Input: part model. Units: mm. Frame: model coordinates. Face numbers are marked on the shaded views. A direction names the side the tool comes from. Round coordinates to 2 decimals unless told otherwise and drop trailing zeros. Write each loop counter-clockwise with the first axis right and the second up, starting at its lowest first coordinate (ties: lowest second). Pieces come first, ordered by that corner, then holes. Notation, with made-up numbers: (84.25, -17) - (108.25, -17) arc R25 ccw to (108.25, 21) - close; hole circle Ø1 at (59, 34). An arc over 180 degrees is marked (long way). One line per item, written item: value. Start each with the question number.
```python
from build123d import *

# Parameters (mm, degrees)
F1_DEPTH = 12.7
F2_W     = 22.225
F2_H     = 12.7
F3_DEPTH = 10.16
F4_R     = 5.08
F5_R     = 3.81
F6_W     = 2.032
F6_H     = 1.016
F7_DEPTH = 1.905
F8_R     = 0.50799


# Not quite as in the source:
# - a fillet or chamfer is up to 0.001 mm smaller than in the source, because OpenCascade refuses the exact size


with BuildPart() as f1:
    # F0 (on Front) → F1 (new body)
    with BuildSketch(Plane.XZ):
        with BuildLine():
            Line((-12.7675240695, 14.3095031442), (-12.7675240695, -11.0904968558))
            Line((-12.7675240695, -11.0904968558), (9.4574759305, -11.0904968558))
            Line((9.4574759305, -11.0904968558), (9.4574759305, 14.3095031442))
            ThreePointArc((9.4574759305, 14.3095031442), (-1.6550240695, 3.1970031442), (-12.7675240695, 14.3095031442))
        make_face()
        with BuildLine():
            ThreePointArc((9.4574759305, 14.3095031442), (-1.6550240695, 25.4220031442), (-12.7675240695, 14.3095031442))
            ThreePointArc((-12.7675240695, 14.3095031442), (-1.6550240695, 3.1970031442), (9.4574759305, 14.3095031442))
        make_face()
    extrude(amount=F1_DEPTH)

    # F2 (on face) → F3 (join)
    with BuildSketch(Plane.XZ.offset(12.7)):
        with Locations((-1.6550240695, -4.7404968558)):
            Rectangle(F2_W, F2_H)
    extrude(amount=F3_DEPTH)

    # F4
    f4_edges = [f1.edges().sort_by_distance(p)[0] for p in [
        (9.457476, -12.7, 7.959503),
        (-12.767524, -17.78, 1.609503),
        (9.457476, -17.78, 1.609503),
    ]]
    fillet(f4_edges, radius=F4_R)

    # F5
    f5_edges = [f1.edges().sort_by_distance(p)[0] for p in [
        (-12.767524, -11.43, -11.090497),
        (9.457476, -11.43, -11.090497),
    ]]
    fillet(f5_edges, radius=F5_R)

    # F6 (on face) → F7 (join)
    with BuildSketch(Plane(origin=(0, 0, 0), x_dir=(-1, 0, 0), z_dir=(0, 1, 0))):
        with Locations((1.6550240695, 14.3095031442)):
            Rectangle(F6_W, F6_H)
    extrude(amount=F7_DEPTH)

    # F8 (radius 0.508 in the source; OpenCascade refuses exactly that, so slightly less here)
    f8_edges = [f1.edges().sort_by_distance(p)[0] for p in [
        (-0.639024, 0.9525, 14.817503),
        (-0.639024, 0.9525, 13.801503),
        (-2.671024, 0.9525, 13.801503),
        (-2.671024, 0.9525, 14.817503),
    ]]
    fillet(f8_edges, radius=F8_R)


solid = f1.part
```
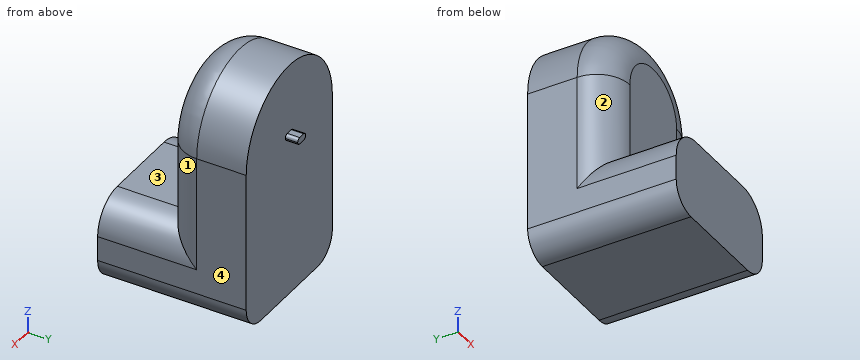
Q1. Cut plane B-B, the plane z = 10. Output: boundary loops of the cut face in (x, y).
Q2. Cut plane D-D, the plane z = -3. Output: boundary loops of the cut face in (x, y).
Q3. Contact query for flat-ended pins moving along their axis: pin 1 Ø3 at (x, z) = (-0.5, 14) entering from -Y; pin 2 Ø6 at (y, z) = (-1.5, 18.5) entering from +X; pin 3 Ø1 at (x, z) = (-1.5, 0) entering from +Y. Output: stop coordinate, or through.
Q4. Material intervals for probe 1 along Z at (x, y) = (-0.25, -21); probe 2 along Y at (x, z) = (8, -6); probe 3 along Y at (x, z) = (-4.25, 20), sorted ascending. Write a range as from..to.
Q5. Cut plane C-C, the plane y = -3. Output: boundary loops of the cut face in (x, z) (1 decimal).
Q6. Access query for the marked faces 1, 2, 3 and 4. Directions: +Z, -Z, +X, -X, +Y, -Y. A direction counts if a zero-diameter tool reaches every point of the face in a straight line with its end or side. Return the directions, or none.
Q7. Cut plane A-A, the plane y = -14.5. Output: boundary loops of the cut face in (x, z), and give its area (3 significant figures).
A:
1. outline: (-12.77, -7.62) arc R5.08 ccw to (-7.69, -12.7) - (4.38, -12.7) arc R5.08 ccw to (9.46, -7.62) - (9.46, 0) - (-12.77, 0) - close
2. outline: (-12.77, -7.62) arc R5.08 ccw to (-12.75, -8.09) - (-12.75, -22.86) - (9.44, -22.86) - (9.44, -8.09) arc R5.08 ccw to (9.46, -7.62) - (9.46, 0) - (-12.77, 0) - close
3. pin 1: stops at y = -12.7
3. pin 2: stops at x = 9.39
3. pin 3: stops at y = 0
4. probe 1: z = -11.09..1.61
4. probe 2: y = -22.86..0
4. probe 3: y = -12.7..0
5. outline: (-12.8, -7.3) arc R3.8 ccw to (-9, -11.1) - (5.6, -11.1) arc R3.8 ccw to (9.5, -7.3) - (9.5, 14.3) arc R11.1 ccw to (-12.8, 14.3) - close
6. face 1: +Z, +X, -Y
6. face 2: +Z, -X, -Y
6. face 3: +Z, +X, -X, -Y
6. face 4: +Z, -Z, +X, +Y, -Y
7. outline: (-12.77, -7.28) arc R3.81 ccw to (-8.96, -11.09) - (5.65, -11.09) arc R3.81 ccw to (9.46, -7.28) - (9.46, -3.47) arc R5.08 ccw to (4.38, 1.61) - (-7.69, 1.61) arc R5.08 ccw to (-12.77, -3.47) - close
7. area: 265 mm²
